Could you check a few things on this model? Use its own coordinates, in mm. A direction names the side the tool comes from. Give positions to 0.01 mm unless a question says otherwise; leave off trailing zeros. Loops run counter-clockwise (first coordinate to the right, second up) from the corner with the lowest first, then second, coordinate; pieces in that order, holes last. Notation, with made-up numbers: (44, 50) - (98, 50) arc R17 ccw to (98, 63) - close; hole circle Ø10 at (-1, 34). An arc over 180 degrees is marked (long way). Answer in a Markdown table with one row per item. Add a question column.
```python
from build123d import *

# Parameters (mm, degrees)
SKETCH1_R           = 69.85
BOSS_EXTRUDE1_DEPTH = 19.05
SKETCH3_R           = 34.925
BOSS_EXTRUDE2_DEPTH = 38.1
BOSS_EXTRUDE2_TAPER = 3
SKETCH4_R           = 19.05
CUT_EXTRUDE1_DEPTH  = 20.05
SKETCH5_R           = 19.05
BOLT_HOLE_DEPTH     = 58.15
SKETCH6_R           = 6.35
CUT_EXTRUDE3_DEPTH  = 20.05
CIRPATTERN2_COUNT   = 4
FILLET1_R           = 6.35
CHAMFER1_SIZE       = 2.032


with BuildPart() as part:
    # Sketch1 → Boss-Extrude1 (new body)
    with BuildSketch(Plane.XY):
        Circle(SKETCH1_R)
    extrude(amount=BOSS_EXTRUDE1_DEPTH)

    # Sketch3 → Boss-Extrude2 (add)
    with BuildSketch(Plane.XY.offset(57.15)):
        Circle(SKETCH3_R)
    extrude(amount=-BOSS_EXTRUDE2_DEPTH, taper=BOSS_EXTRUDE2_TAPER)

    # Sketch4 → Cut-Extrude1 (cut, through all)
    with BuildSketch(Plane.XY.offset(19.05)):
        Circle(SKETCH4_R)
    extrude(amount=-CUT_EXTRUDE1_DEPTH, mode=Mode.SUBTRACT)

    # Sketch5 → Bolt Hole (cut, through all)
    with BuildSketch(Plane.XY.offset(57.15)):
        Circle(SKETCH5_R)
    extrude(amount=-BOLT_HOLE_DEPTH, mode=Mode.SUBTRACT)

    # Sketch6 → Cut-Extrude3 (cut, through all)
    with BuildSketch(Plane.XY.offset(19.05)):
        with Locations((0, 53.975)):
            Circle(SKETCH6_R)
    cut_extrude3 = extrude(amount=-CUT_EXTRUDE3_DEPTH, mode=Mode.SUBTRACT)

    # CirPattern2: Cut-Extrude3 ×4 about axis
    cirpattern2_axis = Axis((0, 0, 0), (0, 0, 1))
    for i in range(1, CIRPATTERN2_COUNT):
        add(cut_extrude3.rotate(cirpattern2_axis, i * 360 / CIRPATTERN2_COUNT), mode=Mode.SUBTRACT)

    # Fillet1
    fillet1_edges = [part.edges().sort_by_distance(p)[0] for p in [
        (-69.85, 0, 19.05),
        (-34.925, 0, 57.15),
        (-32.928263609, 0, 19.05),
    ]]
    fillet(fillet1_edges, radius=FILLET1_R)

    # Chamfer1
    chamfer1_edges = [part.edges().sort_by_distance(p)[0] for p in [
        (-19.05, 0, 57.15),
    ]]
    chamfer(chamfer1_edges, length=CHAMFER1_SIZE)


solid = part.part
```
(1) I want a section at A-A on x = 0. State how many separate pieces and enclosed holes the cut face has, then the cut area to 3 significant figures.
(2) Please list where these lines run through material, in increasing order: line 1 (Z direction, x = 52, y = -33); line 2 (Y direction, x = -7.5, z = 21); line 3 (Y direction, x = -1.5, z = 35.5).
(3) We'd pull the mould along X, two halves only. Please class faces 3 (the cylindrical face through (-48.34, 2.93, 9.66)), 4 (the flat face through (-11, -19, 57.15)), 5 (the conical face through (32.214, 10.145, 35.178)): pulls with the +X half, pulls with the -X half, needs draft (parallel to the pull), parting line crosses it, or undercut.
(4) I want a section at D-D on z = 22. Please give me the cut outline in (x, y), then the cut area to 3 significant figures.
(5) I want a section at B-B on z = 14.5. Please give me the cut outline in (x, y) (3 decimals), then the cut area to 3 significant figures.
(6) For pin 1 Ø8 at (y, z) = (-30, 49.5) entering from -X; pin 2 Ø20.5 at (x, y) = (0, 53.975) entering from +Z; pin 3 Ø10 at (x, y) = (46.5, -50.5) entering from +Z, each with a flat end and sliding along its axis, tell me the tip position at first contact or that it passes through.
(7) On a 3-axis mill with a long thin cutter (end or side, diameter ignored), from which of +Z, -Z, +X, -X, +Y, -Y can I reach the whole of each face in a straight line? I mean faces 1 (the cylindrical face through (-55.431, -42.503, 6.261)), 2 (the flat face through (-29.1, -27.3, 19.05)). Say none if no direction works.
Reported:
| question | item | result |
|---|---|---|
| 1 | separate pieces | 4 |
| 1 | enclosed holes | 0 |
| 1 | area | 2,560 mm² |
| 2 | line 1 | 0 to 19.05 |
| 2 | line 2 | -34.23 to -17.51, 17.51 to 34.23 |
| 2 | line 3 | -33.76 to -18.99, 18.99 to 33.76 |
| 3 | face 3 | undercut |
| 3 | face 4 | needs draft |
| 3 | face 5 | parting line crosses it |
| 4 | outline | circle Ø68.51 at (0, 0); hole circle Ø38.1 at (0, 0) |
| 4 | area | 2,550 mm² |
| 5 | outline | circle Ø139.179 at (0, 0); hole circle Ø12.7 at (-53.975, 0); hole circle Ø38.1 at (0, 0); hole circle Ø12.7 at (0, -53.975); hole circle Ø12.7 at (0, 53.975); hole circle Ø12.7 at (53.975, 0) |
| 5 | area | 13,600 mm² |
| 6 | pin 1 | x = -22.72 |
| 6 | pin 2 | z = 19.05 |
| 6 | pin 3 | z = 19.05 |
| 7 | face 1 | +Z, -Z |
| 7 | face 2 | +Z |
